```python
from build123d import *

# Parameters (mm, degrees)
SKETCH1_W           = 57.15
SKETCH1_H           = 21.59
BOSS_EXTRUDE1_DEPTH = 35.052
SKETCH1_4_W         = 57.15
SKETCH1_4_H         = 21.59
BOSS_EXTRUDE2_DEPTH = 66.802
FILLET1_R           = 9.652
CUT_EXTRUDE1_DEPTH  = 22.59


with BuildPart() as part:
    # Sketch1 → Boss-Extrude1 (new body)
    with BuildSketch(Plane.XY):
        with BuildLine():
            Line((-44.45, 0), (0, 0))
            Line((0, 0), (0, 36.576))
            ThreePointArc((0, 36.576), (-5.579615818, 50.046384182), (-19.05, 55.626))
            Line((-19.05, 55.626), (-93.726, 55.626))
            ThreePointArc((-93.726, 55.626), (-99.293758795, 53.319758795), (-101.6, 47.752))
            Line((-101.6, 47.752), (-101.6, 21.59))
            Line((-101.6, 21.59), (-44.45, 21.59))
            Line((-44.45, 21.59), (-44.45, 0))
        make_face()
        with Locations((-73.025, 10.795)):
            Rectangle(SKETCH1_W, SKETCH1_H)
    extrude(amount=BOSS_EXTRUDE1_DEPTH)

    # Sketch1_4 → Boss-Extrude2 (add)
    with BuildSketch(Plane.XY):
        with Locations((-73.025, 10.795)):
            Rectangle(SKETCH1_4_W, SKETCH1_4_H)
    extrude(amount=BOSS_EXTRUDE2_DEPTH)

    # Fillet1
    fillet1_edges = [part.edges().sort_by_distance(p)[0] for p in [
        (-73.025, 21.59, 35.052),
    ]]
    fillet(fillet1_edges, radius=FILLET1_R)

    # Sketch3 → Cut-Extrude1 (cut, through all)
    with BuildSketch(Plane(origin=(0, 21.59, 0), x_dir=(1, 0, 0), z_dir=(0, 1, 0))):
        Polygon((-83.312, -66.802), (-44.45, -56.642), (-44.45, -66.802), align=None)
    extrude(amount=-CUT_EXTRUDE1_DEPTH, mode=Mode.SUBTRACT)


solid = part.part
```
Input: part model. Units: mm. Frame: model coordinates. A direction names the side the tool comes from. Give positions to 0.01 mm unless a question says otherwise; leave off trailing zeros. Order: outer loops, then holes, each group sorted by start corner. A loop starts at its lowest first (then second) coordinate and runs counter-clockwise, first axis right, second up. Notation, with made-up numbers: M 21,-37.75 L 67,-37.75 A24 cw 67,-19.75 Z; hole C 10,71 d3. An arc over 180 degrees is marked long. One line per question, with ' | ' between items. Start each with the question number.
1. Access query for faces 1 (the face through (-40, 34, 35.052)), 2 (the face through (0, 18, 17)), 3 (the face through (-44.45, 12, 46)), 4 (the face through (-73, 21.59, 53)). Directions: +Z, -Z, +X, -X, +Y, -Y. A direction counts if a zero-diameter tool reaches every point of the face in a straight line with its end or side. Return the directions, or none.
2. Section query B-B (x = -90). Return the cut outline in (y, z).
3. Section query C-C (z = 9.5). Return the cut outline in (x, y).
4. Material intervals for probe 1 along Z at (x, y) = (-66, 47); probe 2 along X at (y, z) = (21.5, 43.5); probe 3 along X at (y, z) = (37, 5), sorted ascending. Write a range as [from, to].
5. First-contact query: pin 1 Ø17.5 at (y, z) = (17.5, 47) entering from +X; pin 2 Ø1.5 at (x, y) = (-30.5, 46) entering from +Z; pin 3 Ø5 at (x, z) = (-32.5, 38) entering from +Y; pin 4 Ø11 at (x, z) = (-71, 54) entering from +Y. Flat tips, straight axial feed; report the tip coordinate or a pass-through.
6. Section query D-D (x = -35). Return the cut outline in (y, z), and give its area (3 significant figures).
7. Section query A-A (y = 13.5). Return the cut outline in (x, z).
Here are the results:
1) face 1: +Z, +X, +Y | face 2: +Z, -Z, +X, +Y, -Y | face 3: +Z, +X, +Y, -Y | face 4: +Z, +X, -X, +Y
2) outline: M 0,0 L 55.63,0 L 55.63,35.05 L 31.24,35.05 A9.65 cw 21.59,44.7 L 21.59,66.8 L 0,66.8 Z
3) outline: M -101.6,0 L 0,0 L 0,36.58 A19.05 ccw -19.05,55.63 L -93.73,55.63 A7.87 ccw -101.6,47.75 Z
4) probe 1: [0, 35.05] | probe 2: [-101.6, -44.45] | probe 3: [-101.6, 0]
5) pin 1: x = -44.45 | pin 2: z = 35.05 | pin 3: through | pin 4: y = 21.59
6) outline: M 0,0 L 55.63,0 L 55.63,35.05 L 0,35.05 Z | area: 1,950 mm²
7) outline: M -101.6,0 L 0,0 L 0,35.05 L -44.45,35.05 L -44.45,56.64 L -83.31,66.8 L -101.6,66.8 Z
